Here's how the part is built. I have some questions about the finished solid (model axes, mm). Coordinates: 2 decimals unless noted, no trailing zeros. Order: outer loops, then holes, each group sorted by start corner. A loop starts at its lowest first (then second) coordinate and runs counter-clockwise, first axis right, second up. Notation, with made-up numbers: (29, 42.5) -> (62, 42.5) arc R21 cw to (62, 63.5) -> close; hole circle Ø8 at (-18.75, 60.25). An arc over 180 degrees is marked (long way). One line per item, written item: value. Start each with the question number.
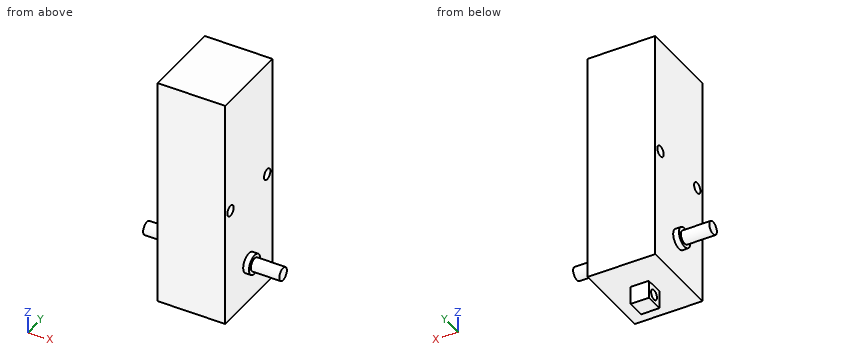
```python
from build123d import *

# Parameters (mm, degrees)
SKETCH1_W               = 64.2
SKETCH1_H               = 22.5
BOSS_EXTRUDE1_DEPTH     = 9.4
SKETCH3_W               = 5
SKETCH3_H               = 5
SKETCH3_R               = 1.4
BOSS_EXTRUDE2_DEPTH     = 2.5
CUT_EXTRUDE1_DEPTH      = 44.129833063
CUT_EXTRUDE1_DEPTH_BACK = 44.129833063
SKETCH4_R               = 1.5


with BuildPart() as part:
    # Sketch1 → Boss-Extrude1 (new, symmetric)
    with BuildSketch(Plane(origin=(0, 0, 0), x_dir=(0, 0, -1), z_dir=(1, 0, 0))):
        Rectangle(SKETCH1_W, SKETCH1_H)
    extrude(amount=BOSS_EXTRUDE1_DEPTH, both=True)

    # Sketch2 → Revolve1 (revolve)
    with BuildSketch(Plane(origin=(0, 0, 0), x_dir=(1, 0, 0), z_dir=(0, 1, 0)), mode=Mode.PRIVATE) as revolve1_sk:
        Polygon((18.9, 20.9), (18.9, 22.7), (11, 22.7), (11, 23.6), (9.4, 23.6), (9.4, 20.9), align=None)
        Polygon((-9.4, 23.6), (-9.4, 20.9), (-18.9, 20.9), (-18.9, 22.7), (-11, 22.7), (-11, 23.6), align=None)
    revolve(revolve1_sk.sketch.rotate(Axis((0, 0, -20.9), (1, 0, 0)), 180), axis=Axis((0, 0, -20.9), (1, 0, 0)))

    # Sketch3 → Boss-Extrude2 (add, symmetric)
    with BuildSketch(Plane(origin=(0, 0, 0), x_dir=(0, 0, -1), z_dir=(1, 0, 0))):
        with Locations((34.6, 0)):
            Rectangle(SKETCH3_W, SKETCH3_H)
        with Locations((34.7, 0)):
            Circle(SKETCH3_R, mode=Mode.SUBTRACT)
    extrude(amount=BOSS_EXTRUDE2_DEPTH, both=True)

    # Sketch4 → Cut-Extrude1 (cut, two sides: drawn at the far end of the back side and taken through both)
    with BuildSketch(Plane(origin=(0, 0, 0), x_dir=(0, 0, -1), z_dir=(1, 0, 0)).offset(-CUT_EXTRUDE1_DEPTH_BACK)):
        with Locations((0.3, 8.75)):
            Circle(SKETCH4_R)
        with Locations((0.3, -8.75)):
            Circle(SKETCH4_R)
    extrude(amount=CUT_EXTRUDE1_DEPTH + CUT_EXTRUDE1_DEPTH_BACK, mode=Mode.SUBTRACT)


solid = part.part
```
Q1. Imagine slicing it at B-B (z = -0.3). Write out the boundary of the cut face in (x, y).
Q2. Imagine slicing it at C-C (y = -8.75). Write out the boundary of the cut face in (x, z), plus the area to 3 significant figures.
Q3. For P1, Ø11, axis at y = 2.5, z = 9.5, coming from the +X side; P2, Ø7, axis at y = -1.5, z = -5.5, coming from the -X side; P3, Ø4, axis at x = 0.5, z = -35, coming from the -Y side, each with a flat end and sliding along its axis, tell me the tip position at first contact or that it passes through.
Q4. Imagine slicing it at A-A (x = 1.5). Write out the boundary of the cut face in (y, z).
Q5. Imagine slicing it at D-D (z = -34.7). Write out the boundary of the cut face in (x, y), plus the area to 3 significant figures.
Q6. I need wall thicknesses on line 1 (Y direction, x = 1, z = -0.3); line 2 (Z direction, x = -0.5, y = 8.75); line 3 (X direction, y = 0.5, z = -8). Which ranges of each line are inside material? Lowest first, please.
Completed:
1. outline: (-9.4, -11.25) -> (9.4, -11.25) -> (9.4, -10.25) -> (-9.4, -10.25) -> close; (-9.4, -7.25) -> (9.4, -7.25) -> (9.4, 7.25) -> (-9.4, 7.25) -> close; (-9.4, 10.25) -> (9.4, 10.25) -> (9.4, 11.25) -> (-9.4, 11.25) -> close
2. outline: (-9.4, -32.1) -> (9.4, -32.1) -> (9.4, -1.8) -> (-9.4, -1.8) -> close; (-9.4, 1.2) -> (9.4, 1.2) -> (9.4, 32.1) -> (-9.4, 32.1) -> close
2. area: 1,150 mm2
3. P1: stops at x = 9.4
3. P2: stops at x = -9.4
3. P3: stops at y = -2.5
4. outline: (-11.25, -32.1) -> (-2.5, -32.1) -> (-2.5, -37.1) -> (2.5, -37.1) -> (2.5, -32.1) -> (11.25, -32.1) -> (11.25, 32.1) -> (-11.25, 32.1) -> close; hole circle Ø3 at (-8.75, -0.3); hole circle Ø2.8 at (0, -34.7); hole circle Ø3 at (8.75, -0.3)
5. outline: (-2.5, -2.5) -> (2.5, -2.5) -> (2.5, -1.4) -> (-2.5, -1.4) -> close; (-2.5, 1.4) -> (2.5, 1.4) -> (2.5, 2.5) -> (-2.5, 2.5) -> close
5. area: 11.0 mm2
6. line 1: y = -11.25 to -10.25, -7.25 to 7.25, 10.25 to 11.25
6. line 2: z = -32.1 to -1.8, 1.2 to 32.1
6. line 3: x = -9.4 to 9.4
